```python
from build123d import *

# Parameters (mm, degrees)
SKETCH1_R           = 5.55625
BOSS_EXTRUDE1_DEPTH = 18.4404
BOSS_EXTRUDE2_DEPTH = 4.2545
SKETCH2_R           = 3.556
CUT_EXTRUDE1_DEPTH  = 39.822706284
FILLET1_R           = 0.762


with BuildPart() as part:
    # Sketch1 → Boss-Extrude1 (new, symmetric)
    with BuildSketch(Plane.XY):
        Circle(SKETCH1_R)
    extrude(amount=BOSS_EXTRUDE1_DEPTH, both=True)

    # Sketch3 → Boss-Extrude2 (add, symmetric)
    with BuildSketch(Plane.XY):
        Polygon((9.165435523, 0), (4.582717762, 7.9375), (-4.582717762, 7.9375), (-9.165435523, 0), (-4.582717762, -7.9375), (4.582717762, -7.9375), align=None)
    extrude(amount=BOSS_EXTRUDE2_DEPTH, both=True)

    # Sketch2 → Cut-Extrude1 (cut, through all)
    with BuildSketch(Plane.XY.offset(18.4404)):
        Circle(SKETCH2_R)
    extrude(amount=-CUT_EXTRUDE1_DEPTH, mode=Mode.SUBTRACT)

    # Fillet1
    fillet1_edges = [part.edges().sort_by_distance(p)[0] for p in [
        (-5.55625, 0, -4.2545),
        (-5.55625, 0, 4.2545),
    ]]
    fillet(fillet1_edges, radius=FILLET1_R)


solid = part.part
```
Input: part model. Units: mm. Frame: model coordinates. A direction names the side the tool comes from. Round coordinates to 2 decimals unless told otherwise and drop trailing zeros. Write each loop counter-clockwise with the first axis right and the second up, starting at its lowest first coordinate (ties: lowest second). Pieces come first, ordered by that corner, then holes. Notation, with made-up numbers: M -26.5,-4.75 L 20.5,-4.75 A12 ccw 20.5,2.25 Z; hole C 53,57.25 d4. An arc over 180 degrees is marked long. Write each question's results on one line, items separated by ' | '.
Q1. Pin query (flat end, axial travel): P1, Ø6, axis at y = -0.5, z = -13, coming from the -X side; P2, Ø1.5, axis at y = 1.5, z = 10.5, coming from the -X side; P3, Ø4, axis at x = 0, z = -13.5, coming from the +Y side. Return the tip coordinate at first contact, or that it passes through.
Results:
P1: stops at x = -5.56 | P2: stops at x = -5.51 | P3: stops at y = 5.56
Q2. Section query A-A (x = 0). Return loops of the section in (y, z), and give its area (3 significant figures).
Results:
outline: M -7.94,-4.25 L -6.32,-4.25 A0.76 cw -5.56,-5.02 L -5.56,-18.44 L -3.56,-18.44 L -3.56,18.44 L -5.56,18.44 L -5.56,5.02 A0.76 cw -6.32,4.25 L -7.94,4.25 Z; M 3.56,-18.44 L 5.56,-18.44 L 5.56,-5.02 A0.76 cw 6.32,-4.25 L 7.94,-4.25 L 7.94,4.25 L 6.32,4.25 A0.76 cw 5.56,5.02 L 5.56,18.44 L 3.56,18.44 Z | area: 189 mm^2
Q3. Line query: line 1 along Y through (x, z) = (0, -10); line 2 along Y through (x, z) = (0, 2.5); line 3 along Z through (x, y) = (1, 7). Output: solid intervals per line, ascending.
Results:
line 1: y = -5.56 to -3.56, 3.56 to 5.56 | line 2: y = -7.94 to -3.56, 3.56 to 7.94 | line 3: z = -4.25 to 4.25
Q4. Section query B-B (z = 16). Return loops of the section in (x, y), and give its area (3 significant figures).
Results:
outline: C 0,0 d11.11; hole C 0,0 d7.11 | area: 57.3 mm^2
Q5. Draft query along X for faces 4 (the face through (6.842, -4.024, 0.06)), 5 (the face through (-0.77, -3.47, 0.26)), 6 (the face through (0, -4, 18.44)). Return one class per face: released by +X, released by -X, zero draft, split by the parting line, or undercut.
Results:
face 4: released by +X | face 5: undercut | face 6: zero draft
Q6. Access query for faces 1 (the face through (5.3, 1.67, 11.82)), 2 (the face through (5.4, 3.6, -4.254)), 3 (the face through (-6.842, 4.024, 0.06)). Directions: +Z, -Z, +X, -X, +Y, -Y. A direction counts if a zero-diameter tool reaches every point of the face in a straight line with its end or side. Return the directions, or none.
Results:
face 1: +Z | face 2: -Z | face 3: +Z, -Z, -X, +Y
Q7. Section query C-C (x = 7). Return loops of the section in (y, z), and give its area (3 significant figures).
Results:
outline: M -3.75,-4.25 L 3.75,-4.25 L 3.75,4.25 L -3.75,4.25 Z | area: 63.8 mm^2
